Design review of the part built by this model. Coordinates are the model's own, in mm. A direction names the side the tool comes from. Round coordinates to 2 decimals unless told otherwise and drop trailing zeros. Loops run counter-clockwise (first coordinate to the right, second up) from the corner with the lowest first, then second, coordinate; pieces in that order, holes last. Notation, with made-up numbers: (-36, 67) - (-7, 67) arc R32 ccw to (-7, 103) - close; hole circle Ø1 at (48, 6). An arc over 180 degrees is marked (long way). Return JSON: item names as keys, results as strings. Group by question number.
Autodesk Fusion 360 part; units mm, degrees
sketch "Sketch1" plane through (0, 0, 0) normal (1, 0, 0) x (0, 1, 0)
  circle A0 centre (0, 0) radius 19.5
  dimension "d1" = 39
extrude "Extrude1" add sketch "Sketch1" along normal blind 10
sketch "Sketch2" plane through (0, 0, 0) normal (1, 0, 0) x (0, 1, 0)
  line L0 (5.8998, 1.1158) -> (1.9836, 5.6673)
  line L1 (1.9836, 5.6673) -> (-3.9163, 4.5515)
  line L2 (-3.9163, 4.5515) -> (-5.8998, -1.1158)
  line L3 (-5.8998, -1.1158) -> (-1.9836, -5.6673)
  line L4 (-1.9836, -5.6673) -> (3.9163, -4.5515)
  line L5 (3.9163, -4.5515) -> (5.8998, 1.1158)
  dimension "d4" = 5.2
extrude "Extrude2" cut sketch "Sketch2" along normal blind 4.2
sketch "Sketch3" plane through (10, 0, 0) normal (1, 0, 0) x (0, 1, 0)
  circle A0 centre (0, 0) radius 19.5
  circle A1 centre (0, 0) radius 10.5
  dimension "d7" = 21
extrude "Extrude3" cut sketch "Sketch3" against normal blind 2.6 contours A1
sketch "Sketch4" plane through (0, 0, 0) normal (1, 0, 0) x (0, 1, 0)
sketch "Sketch5" plane through (0, 0, 0) normal (1, 0, 0) x (0, 1, 0)
  circle A0 centre (0, -15) radius 1.5
  dimension "d10" = 3
sketch "Sketch6" plane through (0, 0, 0) normal (1, 0, 0) x (0, 1, 0)
  circle A0 centre (-14, 0) radius 1.5
  circle A1 centre (0, 14) radius 1.5
  circle A2 centre (14, 0) radius 1.5
  dimension "d13" = 3
  dimension "d14" = 3
  dimension "d15" = 3
sketch "Sketch7" plane through (0, 0, 0) normal (-1, 0, 0) x (0, -1, 0)
  line L0 (1.9836, -5.6673) -> (-3.9163, -4.5515)
  line L1 (-3.9163, -4.5515) -> (-5.8998, 1.1158)
  line L2 (-5.8998, 1.1158) -> (-1.9836, 5.6673)
  line L3 (-1.9836, 5.6673) -> (3.9163, 4.5515)
  line L4 (3.9163, 4.5515) -> (5.8998, -1.1158)
  line L5 (5.8998, -1.1158) -> (1.9836, -5.6673)
  circle A0 centre (0, 0) radius 19.5
  circle A1 centre (0, 15) radius 1.5
  circle A2 centre (-15, 0) radius 1.5
  point P0 (-15, 0)
  dimension "d18" = 3
  dimension "d28" = 3
sketch "Sketch8" plane through (0, 0, 0) normal (1, 0, 0) x (0, 1, 0)
  circle A0 centre (-15, 0) radius 1.5
  dimension "d21" = 3
extrude "Extrude7" cut sketch "Sketch8" along normal blind 12
extrude "Extrude8" cut sketch "Sketch5" along normal blind 15
extrude "Extrude9" cut sketch "Sketch7" against normal blind 15 contours A1
extrude "Extrude10" cut sketch "Sketch7" against normal blind 15 contours A2
sketch "Sketch10" plane through (7.4, 0, 0) normal (1, 0, 0) x (0, 1, 0)
  circle A0 centre (0, 0) radius 10.5
  line L0 (-3.003, -16.7268) -> (-0.0431, -18.5265)
  line L1 (-0.0431, -18.5265) -> (2.9955, -16.8631)
  line L2 (2.9955, -16.8631) -> (3.0742, -13.3999)
  line L3 (3.0742, -13.3999) -> (0.1143, -11.6001)
  line L4 (0.1143, -11.6001) -> (-2.9243, -13.2636)
  line L5 (-2.9243, -13.2636) -> (-3.003, -16.7268)
  point P0 (0.0356, -15.0633)
  dimension "d32" = 3
extrude "Extrude11" cut sketch "Sketch10" along normal blind 2600 contours L0 L1 L2 L3 L4 L5
sketch "Sketch11" plane through (7.4, 0, 0) normal (1, 0, 0) x (0, 1, 0)
  circle A0 centre (0, 0) radius 10.5
  line L0 (-18, -1.7321) -> (-15, -3.4641)
  line L1 (-15, -3.4641) -> (-12, -1.7321)
  line L2 (-12, -1.7321) -> (-12, 1.7321)
  line L3 (-12, 1.7321) -> (-15, 3.4641)
  line L4 (-15, 3.4641) -> (-18, 1.7321)
  line L5 (-18, 1.7321) -> (-18, -1.7321)
  point P0 (-15, 0)
  dimension "d35" = 3
extrude "Extrude12" cut sketch "Sketch11" along normal blind 2.6 contours L0 L1 L2 L3 L4 L5
sketch "Sketch13" plane through (7.4, 0, 0) normal (1, 0, 0) x (0, 1, 0)
  circle A0 centre (0, 0) radius 10.5
  line L0 (3, 16.7321) -> (0, 18.4641)
  line L1 (0, 18.4641) -> (-3, 16.7321)
  line L2 (-3, 16.7321) -> (-3, 13.2679)
  line L3 (-3, 13.2679) -> (0, 11.5359)
  line L4 (0, 11.5359) -> (3, 13.2679)
  line L5 (3, 13.2679) -> (3, 16.7321)
  point P0 (0, 15)
  dimension "d39" = 3
extrude "Extrude13" cut sketch "Sketch13" along normal blind 2.6 contours L0 L1 L2 L3 L4 L5
sketch "Sketch14" plane through (7.4, 0, 0) normal (1, 0, 0) x (0, 1, 0)
  circle A0 centre (0, 0) radius 10.5
  line L0 (12, -1.7321) -> (15, -3.4641)
  line L1 (15, -3.4641) -> (18, -1.7321)
  line L2 (18, -1.7321) -> (18, 1.7321)
  line L3 (18, 1.7321) -> (15, 3.4641)
  line L4 (15, 3.4641) -> (12, 1.7321)
  line L5 (12, 1.7321) -> (12, -1.7321)
  point P0 (15, 0)
extrude "Extrude14" cut sketch "Sketch14" along normal blind 2.6 contours L0 L1 L2 L3 L4 L5
sketch "Sketch15" plane through (7.4, 0, 0) normal (1, 0, 0) x (0, 1, 0)
Q1. Tool access review of faces 1 (the cylindrical face through (3.65, 16.5, 0.07)), 2 (the flat face through (8.68, 1.45, -17.71)), 3 (the flat face through (2.071, 4.894, -1.758)): name each direction out of +Z, -Z, +X, -X, +Y, -Y from which nothing blocks a thin tool from reaching the whole face with its end or side.
Q2. For line 1 (Z direction, x = 5.75, y = 0); line 2 (Z direction, x = 2, y = 0); line 3 (Y direction, x = 2.5, z = 1), list the stretches that pass through material, from the lowest coordinate up.
Q3. Add section A-A, the plane x = 8. State the section outline as (y, z) points, plus the area to 3 significant figures.
Q4. Add section C-C, the plane z = -15. State the section outline as (x, y) points, plus the area to 3 significant figures.
Q5. Add section B-B, the plane z = 0. State the section outline as (x, y) points, plus the area to 3 significant figures.
Q6. Add section D-D, the plane z = -8. State the section outline as (x, y) points.
Q7. Insertion check: pin 1 Ø17 at (y, z) = (0, -0.5) entering from +X; pin 2 Ø3 at (x, z) = (9, 15.5) entering from -Y; pin 3 Ø1 at (x, y) = (4.5, 12.5) entering from -Z. Each pin has a flat end and moves straight along its axis. Give the tip position at first contact, or say it passes through.
Evaluation:
{
 "1": {"face 1": "+X, -X", "face 2": "+X", "face 3": "-X"},
 "2": {"line 1": "-19.5 to -16.5, -13.5 to 13.5, 16.5 to 19.5", "line 2": "-19.5 to -16.5, -13.5 to -5.29, 5.29 to 13.5, 16.5 to 19.5", "line 3": "-19.47 to -16.12, -13.88 to -5.16, 5.86 to 13.88, 16.12 to 19.47"},
 "3": {"outline": "circle Ø39 at (0, 0); hole (-18, -1.73) - (-15, -3.46) - (-12, -1.73) - (-12, 1.73) - (-15, 3.46) - (-18, 1.73) - close; hole circle Ø21 at (0, 0); hole (-3, -16.73) - (-0.04, -18.53) - (3, -16.86) - (3.07, -13.4) - (0.11, -11.6) - (-2.92, -13.26) - close; hole (-3, 13.27) - (0, 11.54) - (3, 13.27) - (3, 16.73) - (0, 18.46) - (-3, 16.73) - close; hole (12, -1.73) - (15, -3.46) - (18, -1.73) - (18, 1.73) - (15, 3.46) - (12, 1.73) - close", "area": "724 mm²"},
 "4": {"outline": "(0, -12.46) - (10, -12.46) - (10, -2.96) - (7.4, -2.96) - (7.4, -1.5) - (0, -1.5) - close; (0, 1.5) - (7.4, 1.5) - (7.4, 3.04) - (10, 3.04) - (10, 12.46) - (0, 12.46) - close", "area": "211 mm²"},
 "5": {"outline": "(0, -19.5) - (10, -19.5) - (10, -18) - (7.4, -18) - (7.4, -16.5) - (0, -16.5) - close; (0, -13.5) - (7.4, -13.5) - (7.4, -12) - (10, -12) - (10, -10.5) - (7.4, -10.5) - (7.4, 10.5) - (10, 10.5) - (10, 12) - (7.4, 12) - (7.4, 13.5) - (0, 13.5) - (0, 5.51) - (4.2, 5.51) - (4.2, -5.51) - (0, -5.51) - close; (0, 16.5) - (7.4, 16.5) - (7.4, 18) - (10, 18) - (10, 19.5) - (0, 19.5) - close", "area": "214 mm²"},
 "6": {"outline": "(0, -17.78) - (10, -17.78) - (10, -6.8) - (7.4, -6.8) - (7.4, 6.8) - (10, 6.8) - (10, 17.78) - (0, 17.78) - close"},
 "7": {"pin 1": "x = 7.4", "pin 2": "y = -13.57", "pin 3": "z = -15.37"}
}
